from build123d import *

# Parameters (mm, degrees)
SKETCH2_W               = 90
SKETCH2_H               = 70
BOSS_EXTRUDE1_DEPTH     = 35
SKETCH4_R               = 8
BOSS_EXTRUDE2_DEPTH     = 14
SKETCH6_W               = 6.6
SKETCH6_H               = 5.7
BOSS_EXTRUDE3_DEPTH     = 10
SKETCH10_W              = 6.6
SKETCH10_H              = 5.7
BOSS_EXTRUDE4_DEPTH     = 10
SKETCH7_W               = 6.6
SKETCH7_H               = 5.7
BOSS_EXTRUDE5_DEPTH     = 10
CUT_EXTRUDE1_DEPTH      = 123.786908504
CUT_EXTRUDE1_DEPTH_BACK = 123.786908504
SKETCH11_R              = 1.25
CUT_EXTRUDE2_DEPTH      = 123.786908504
CUT_EXTRUDE2_DEPTH_BACK = 123.786908504
SKETCH15_R              = 1.25
CUT_EXTRUDE3_DEPTH      = 123.786908504
CUT_EXTRUDE3_DEPTH_BACK = 123.786908504
SKETCH14_R              = 1.25
CUT_EXTRUDE4_DEPTH      = 123.786908504
CUT_EXTRUDE4_DEPTH_BACK = 123.786908504
SKETCH12_R              = 1.25
SKETCH16_W              = 6
SKETCH16_H              = 33
CUT_EXTRUDE5_DEPTH      = 33.3
SKETCH19_W              = 6
SKETCH19_H              = 33
CUT_EXTRUDE6_DEPTH      = 33.3
SKETCH18_W              = 6
SKETCH18_H              = 6
CUT_EXTRUDE7_DEPTH      = 33.3
SKETCH17_W              = 6
SKETCH17_H              = 20
CUT_EXTRUDE8_DEPTH      = 33.3
SKETCH20_W              = 25.8
SKETCH20_H              = 17.9
BOSS_EXTRUDE6_DEPTH     = 39.4
SKETCH27_R              = 9
BOSS_EXTRUDE7_DEPTH     = 3
SKETCH29_W              = 2.1
SKETCH29_H              = 25.8
CUT_EXTRUDE14_DEPTH     = 2.5
SKETCH34_W              = 2.1
SKETCH34_H              = 15.4
CUT_EXTRUDE15_DEPTH     = 2.5
SKETCH35_W              = 2.1
SKETCH35_H              = 23.3
CUT_EXTRUDE16_DEPTH     = 2.5
SKETCH36_W              = 2.1
SKETCH36_H              = 12.9
CUT_EXTRUDE17_DEPTH     = 2.5
SKETCH38_R              = 1.875
BOSS_EXTRUDE8_DEPTH     = 20


with BuildPart() as part:
    # Sketch2 → Boss-Extrude1 (new body)
    with BuildSketch(Plane(origin=(0, 0, 0), x_dir=(1, 0, 0), z_dir=(0, 1, 0))):
        with Locations((45, 35)):
            Rectangle(SKETCH2_W, SKETCH2_H)
    extrude(amount=BOSS_EXTRUDE1_DEPTH)

    # Sketch4 → Boss-Extrude2 (add)
    with BuildSketch(Plane.XY):
        with Locations(Location((45, -2.57, 0), (0, 0, 161.261463564))):
            Circle(SKETCH4_R)
    extrude(amount=BOSS_EXTRUDE2_DEPTH)

    # Sketch6 → Boss-Extrude3 (add)
    with BuildSketch(Plane(origin=(0, 0, 0), x_dir=(-1, 0, 0), z_dir=(0, -1, 0))):
        with Locations((-81.82, 55.55)):
            Rectangle(SKETCH6_W, SKETCH6_H)
    extrude(amount=BOSS_EXTRUDE3_DEPTH)

    # Sketch10 → Boss-Extrude4 (add)
    with BuildSketch(Plane.XZ):
        with Locations((81.82, -37.25)):
            Rectangle(SKETCH10_W, SKETCH10_H)
    extrude(amount=BOSS_EXTRUDE4_DEPTH)

    # Sketch7 → Boss-Extrude5 (add)
    with BuildSketch(Plane.XZ):
        with Locations((81.82, -19.65)):
            Rectangle(SKETCH7_W, SKETCH7_H)
    extrude(amount=BOSS_EXTRUDE5_DEPTH)

    # Sketch11 → Cut-Extrude1 (cut, two sides: drawn at the far end of the back side and taken through both)
    with BuildSketch(Plane(origin=(0, 35, 0), x_dir=(1, 0, 0), z_dir=(0, 1, 0)).offset(-CUT_EXTRUDE1_DEPTH_BACK)):
        with Locations(Location((87.55, 2.29, 0), (0, 0, 90))):
            Circle(SKETCH11_R)
    extrude(amount=CUT_EXTRUDE1_DEPTH + CUT_EXTRUDE1_DEPTH_BACK, mode=Mode.SUBTRACT)

    # Sketch15 → Cut-Extrude2 (cut, two sides: drawn at the far end of the back side and taken through both)
    with BuildSketch(Plane(origin=(0, 35, 0), x_dir=(1, 0, 0), z_dir=(0, 1, 0)).offset(-CUT_EXTRUDE2_DEPTH_BACK)):
        with Locations(Location((2.61, 67.35, 0), (0, 0, 90))):
            Circle(SKETCH15_R)
    extrude(amount=CUT_EXTRUDE2_DEPTH + CUT_EXTRUDE2_DEPTH_BACK, mode=Mode.SUBTRACT)

    # Sketch14 → Cut-Extrude3 (cut, two sides: drawn at the far end of the back side and taken through both)
    with BuildSketch(Plane(origin=(0, 35, 0), x_dir=(1, 0, 0), z_dir=(0, 1, 0)).offset(-CUT_EXTRUDE3_DEPTH_BACK)):
        with Locations(Location((2.63, 2.25, 0), (0, 0, 90))):
            Circle(SKETCH14_R)
    extrude(amount=CUT_EXTRUDE3_DEPTH + CUT_EXTRUDE3_DEPTH_BACK, mode=Mode.SUBTRACT)

    # Sketch12 → Cut-Extrude4 (cut, two sides: drawn at the far end of the back side and taken through both)
    with BuildSketch(Plane(origin=(0, 35, 0), x_dir=(1, 0, 0), z_dir=(0, 1, 0)).offset(-CUT_EXTRUDE4_DEPTH_BACK)):
        with Locations(Location((87.71, 67.37, 0), (0, 0, 90))):
            Circle(SKETCH12_R)
    extrude(amount=CUT_EXTRUDE4_DEPTH + CUT_EXTRUDE4_DEPTH_BACK, mode=Mode.SUBTRACT)

    # Sketch16 → Cut-Extrude5 (cut)
    with BuildSketch(Plane(origin=(0, 35, 0), x_dir=(1, 0, 0), z_dir=(0, 1, 0))):
        with Locations((3, 53.5)):
            Rectangle(SKETCH16_W, SKETCH16_H)
    extrude(amount=-CUT_EXTRUDE5_DEPTH, mode=Mode.SUBTRACT)

    # Sketch19 → Cut-Extrude6 (cut)
    with BuildSketch(Plane(origin=(0, 35, 0), x_dir=(1, 0, 0), z_dir=(0, 1, 0))):
        with Locations((3, 16.5)):
            Rectangle(SKETCH19_W, SKETCH19_H)
    extrude(amount=-CUT_EXTRUDE6_DEPTH, mode=Mode.SUBTRACT)

    # Sketch18 → Cut-Extrude7 (cut)
    with BuildSketch(Plane(origin=(0, 35, 0), x_dir=(1, 0, 0), z_dir=(0, 1, 0))):
        with Locations((87, 3)):
            Rectangle(SKETCH18_W, SKETCH18_H)
    extrude(amount=-CUT_EXTRUDE7_DEPTH, mode=Mode.SUBTRACT)

    # Sketch17 → Cut-Extrude8 (cut)
    with BuildSketch(Plane(origin=(0, 35, 0), x_dir=(1, 0, 0), z_dir=(0, 1, 0))):
        with Locations((87, 60)):
            Rectangle(SKETCH17_W, SKETCH17_H)
    extrude(amount=-CUT_EXTRUDE8_DEPTH, mode=Mode.SUBTRACT)

    # Sketch20 → Boss-Extrude6 (add)
    with BuildSketch(Plane(origin=(0, 0, 0), x_dir=(0, 0, -1), z_dir=(1, 0, 0))):
        with Locations((37.6, -4.95)):
            Rectangle(SKETCH20_W, SKETCH20_H)
    extrude(amount=-BOSS_EXTRUDE6_DEPTH)

    # Sketch27 → Boss-Extrude7 (add)
    with BuildSketch(Plane.XY.offset(14)):
        with Locations((45, -2.57)):
            Circle(SKETCH27_R)
    extrude(amount=BOSS_EXTRUDE7_DEPTH)

    # Sketch29 → Cut-Extrude14 (cut)
    with BuildSketch(Plane(origin=(0, 4, 0), x_dir=(1, 0, 0), z_dir=(0, 1, 0))):
        with Locations((-13.05, 37.6)):
            Rectangle(SKETCH29_W, SKETCH29_H)
    extrude(amount=-CUT_EXTRUDE14_DEPTH, mode=Mode.SUBTRACT)

    # Sketch34 → Cut-Extrude15 (cut)
    with BuildSketch(Plane.XY.offset(-24.7)):
        with Locations((-13.05, -6.2)):
            Rectangle(SKETCH34_W, SKETCH34_H)
    extrude(amount=-CUT_EXTRUDE15_DEPTH, mode=Mode.SUBTRACT)

    # Sketch35 → Cut-Extrude16 (cut)
    with BuildSketch(Plane.XZ.offset(13.9)):
        with Locations((-13.05, -38.85)):
            Rectangle(SKETCH35_W, SKETCH35_H)
    extrude(amount=-CUT_EXTRUDE16_DEPTH, mode=Mode.SUBTRACT)

    # Sketch36 → Cut-Extrude17 (cut)
    with BuildSketch(Plane(origin=(0, 0, -50.5), x_dir=(-1, 0, 0), z_dir=(0, 0, -1))):
        with Locations((13.05, -4.95)):
            Rectangle(SKETCH36_W, SKETCH36_H)
    extrude(amount=-CUT_EXTRUDE17_DEPTH, mode=Mode.SUBTRACT)

    # Sketch38 → Boss-Extrude8 (add)
    with BuildSketch(Plane(origin=(0, 0, -70), x_dir=(-1, 0, 0), z_dir=(0, 0, -1))):
        with Locations(Location((-56, 26.2, 0), (0, 0, 180))):
            Circle(SKETCH38_R)
        with Locations(Location((-10, 26.2, 0), (0, 0, 180))):
            Circle(SKETCH38_R)
    extrude(amount=BOSS_EXTRUDE8_DEPTH)


solid = part.part
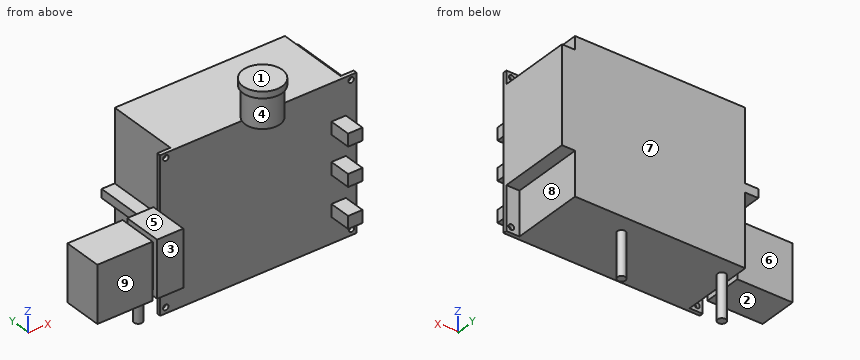
Read the model definition and answer for the solid it produces. Units are mm, in the model's axes. Face numbers are marked on the shaded views. A direction names the side the tool comes from. Give positions to 0.01 mm unless a question says otherwise; leave off trailing zeros. Loops run counter-clockwise (first coordinate to the right, second up) from the corner with the lowest first, then second, coordinate; pieces in that order, holes last. Notation, with made-up numbers: (34, 73.5) -> (63, 73.5) arc R31 ccw to (63, 103.5) -> close; hole circle Ø1 at (-31, -20). An arc over 180 degrees is marked (long way). Use a Markdown table: item, result.
Q1. Section D-D, the plane y = -4.5 is taken. Count the separate pieces of the cut face and the enclosed holes in it, then the cut area to 3 significant figures.
Solved:
| item | result |
|---|---|
| separate pieces | 5 |
| enclosed holes | 0 |
| area | 1,390 mm^2 |
Q2. Section C-C, the plane z = -46.5 is taken. Determine the outline of the cut face in (x, y).
Solved:
| item | result |
|---|---|
| outline | (-39.4, -13.9) -> (-14.1, -13.9) -> (-14.1, -11.4) -> (-12, -11.4) -> (-12, -13.9) -> (0, -13.9) -> (0, 0) -> (90, 0) -> (90, 35) -> (6, 35) -> (6, 1.7) -> (0, 1.7) -> (0, 4) -> (-12, 4) -> (-12, 1.5) -> (-14.1, 1.5) -> (-14.1, 4) -> (-39.4, 4) -> close |
Q3. Determine the mould class of the marked faces 1, 2, 3 and 4 for opening direction Z: pulls with the +Z half, pulls with the -Z half, needs draft (parallel to the pull), parting line crosses it, or undercut.
Solved:
| item | result |
|---|---|
| face 1 | pulls with the +Z half |
| face 2 | pulls with the -Z half |
| face 3 | needs draft |
| face 4 | undercut |
Q4. Section A-A, the plane y = 26.2 is taken. Determine the outline of the cut face in (x, z) (3 decimals), then the cut area to 3 significant figures.
Solved:
| item | result |
|---|---|
| outline | (0, -37) -> (6, -37) -> (6, -70) -> (8.125, -70) -> (8.125, -90) -> (11.875, -90) -> (11.875, -70) -> (54.125, -70) -> (54.125, -90) -> (57.875, -90) -> (57.875, -70) -> (84, -70) -> (84, -50) -> (90, -50) -> (90, -6) -> (84, -6) -> (84, 0) -> (6, 0) -> (6, -33) -> (0, -33) -> close |
| area | 5,900 mm^2 |
Q5. Each of these flat-tipped pins is pushed along its axis until it touches: pin 1 (12 mm diameter, centred on x = 0, z = -71, fed in from -Y); pin 2 (10 mm diameter, centred on y = 24, z = -10, fed in from -X); pin 3 (2 mm diameter, centred on x = 82.5, y = -7, fed in from -Z). Where does it stop, or does it pass through?
Solved:
| item | result |
|---|---|
| pin 1 | stops at y = 0 |
| pin 2 | stops at x = 6 |
| pin 3 | stops at z = -58.4 |
Q6. Section B-B, the plane x = 45 is taken. Determine the outline of the cut face in (y, z), then the cut area to 3 significant figures.
Solved:
| item | result |
|---|---|
| outline | (-11.57, 14) -> (-10.57, 14) -> (-10.57, 0) -> (0, 0) -> (0, -70) -> (35, -70) -> (35, 0) -> (5.43, 0) -> (5.43, 14) -> (6.43, 14) -> (6.43, 17) -> (-11.57, 17) -> close |
| area | 2,730 mm^2 |
Q7. A tool of negligible diameter and unlimited length cuts with its end or side. For the marked faces 5, 6, 7, 8 and 9, from which of +Z, -Z, +X, -X, +Y, -Y can it reach the whole face along a straight path? Write none if from no direction.
Solved:
| item | result |
|---|---|
| face 5 | +Z, -X, +Y, -Y |
| face 6 | +Z, -Z, -X, +Y |
| face 7 | +Z, -Z, +X, -X, +Y |
| face 8 | -Z, +X, +Y |
| face 9 | +Z, -Z, +X, -X, -Y |
Q8. Find the intervals of material crossed by line 1 along X through (y, z) = (0.45, -67.37); line 2 along X through (y, z) = (1.35, -2.29); line 3 along Z through (x, y) = (87.55, 0.7), in increasing order.
Solved:
| item | result |
|---|---|
| line 1 | x = 0 to 1.36, 3.86 to 86.46, 88.96 to 90 |
| line 2 | x = 0 to 1.38, 3.88 to 86.3, 88.8 to 90 |
| line 3 | z = -70 to -68.61, -66.13 to -3.54, -1.04 to 0 |
